The listing builds one solid part. Answer for the finished solid, in the listing's coordinates (mm). Face numbers are marked on the shaded views. A direction names the side the tool comes from. Round coordinates to 2 decimals unless told otherwise and drop trailing zeros. Put each result on its own line as item: value. Start each with the question number.
1. Each of these flat-tipped pins is pushed along its axis until it touches: pin 1 Ø5 at (y, z) = (-7.5, -58.5) entering from +X; pin 2 Ø2 at (x, z) = (28, 4.5) entering from -Y; pin 3 Ø1.5 at (x, z) = (2, -29.5) entering from -Y. Where does it stop, or does it pass through?
2. The mould has two halves that part along Y. Classify the marked faces 1, 2 and 3: +Y half, -Y half, draft (parallel to the pull), parting line (faces both ways), or undercut.
3. Which of the six approach directions +Z, -Z, +X, -X, +Y, -Y give full straight-line access (tool end or side, diameter ignored) to the marked faces 4 and 5?
4. Consider line 1 (Y direction, x = 7.5, z = 0); line 2 (Y direction, x = -1.5, z = 0); line 3 (Z direction, x = -7.5, y = 15). Determine where each line is inside the solid, lowest interval first.
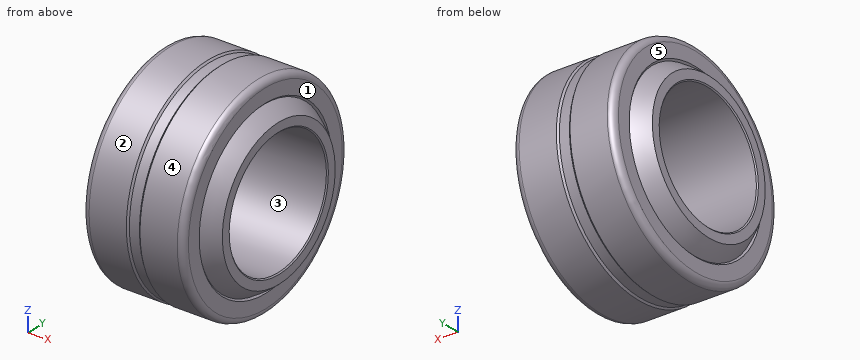
from build123d import *


with BuildPart() as part:
    # Sketch1 → Revolve1 (revolve)
    with BuildSketch(Plane.XY, mode=Mode.PRIVATE) as revolve1_sk:
        with BuildLine():
            Line((-45.212, 51.464994612), (-45.212, 45.241385071))
            Line((-45.212, 45.241385071), (-44.420614929, 44.45))
            Line((-44.420614929, 44.45), (44.420614929, 44.45))
            Line((44.420614929, 44.45), (45.212, 45.241385071))
            Line((45.212, 45.241385071), (45.212, 51.464994612))
            ThreePointArc((45.212, 51.464994612), (40.048905798, 55.577475283), (34.513977442, 59.173946763))
            Line((34.513977442, 59.173946763), (35.7124, 60.372369321))
            Line((35.7124, 60.372369321), (35.7124, 70.14845))
            ThreePointArc((35.7124, 70.14845), (34.404910027, 73.305010027), (31.24835, 74.6125))
            Line((31.24835, 74.6125), (4.843974298, 74.6125))
            Line((4.843974298, 74.6125), (3.57124, 73.4933125))
            Line((3.57124, 73.4933125), (-3.57124, 73.4933125))
            Line((-3.57124, 73.4933125), (-4.843974298, 74.6125))
            Line((-4.843974298, 74.6125), (-31.24835, 74.6125))
            ThreePointArc((-31.24835, 74.6125), (-34.404910027, 73.305010027), (-35.7124, 70.14845))
            Line((-35.7124, 70.14845), (-35.7124, 60.372369321))
            Line((-35.7124, 60.372369321), (-34.513977442, 59.173946763))
            ThreePointArc((-34.513977442, 59.173946763), (-40.048905798, 55.577475283), (-45.212, 51.464994612))
        make_face()
    revolve(revolve1_sk.sketch.rotate(Axis((-45.212, 0, 0), (1, 0, 0)), 270), axis=Axis((-45.212, 0, 0), (1, 0, 0)))


solid = part.part
Resolved:
1. pin 1: x = 38.77
1. pin 2: y = -74.53
1. pin 3: y = -67.64
2. face 1: draft
2. face 2: parting line
2. face 3: undercut
3. face 4: +X, -X
3. face 5: -X
4. line 1: -74.61 to -44.45, 44.45 to 74.61
4. line 2: -73.49 to -44.45, 44.45 to 73.49
4. line 3: -73.09 to -41.84, 41.84 to 73.09
